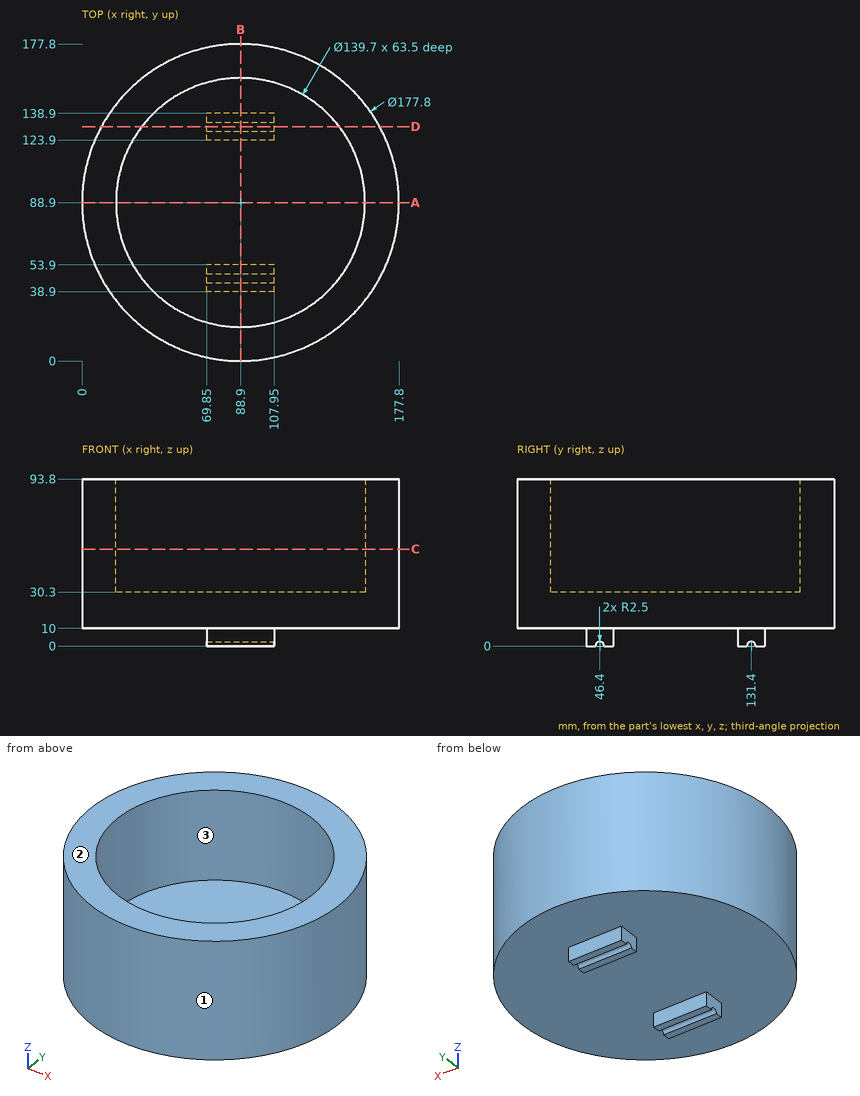
Here's the drawing with two shaded views (mm, measured from the low corner). I have some questions. Round coordinates to 2 decimals unless told otherwise and drop trailing zeros. Order: outer loops, then holes, each group sorted by start corner. A loop starts at its lowest first (then second) coordinate and runs counter-clockwise, first axis right, second up. Notation, with made-up numbers: (8, 89.25) -> (44, 89.25) arc R17 cw to (44, 99.25) -> close; hole circle Ø10 at (35.25, 23). An arc over 180 degrees is marked (long way). Use a Markdown table: item, result. Add a question column.
(1) Suppose I cut it at C-C, the plane z = 54.5. Please give me the cut outline in (x, y), and give its area (3 significant figures).
(2) Suppose I cut it at D-D, the plane y = 131.4. Please give me the cut outline in (x, z), and give its area (3 significant figures).
(3) Suppose I cut it at B-B, the plane x = 88.9. Please give me the cut outline in (y, z), and give its area (3 significant figures).
(4) I need wall thicknesses on line 1 along Y through (x, z) = (88, 62); line 2 along Z through (x, y) = (46.5, 43); line 3 along Y through (x, z) = (60, 79). Which ranges of each line are inside material? Lowest first, please.
(5) If we mould it in two halves opening along Y, with no side actions, what happens to the marked faces 1, 2 and 3? For each: released by +Y, released by -Y, zero draft, split by the parting line, or undercut.
(6) For pin 1 Ø8 at (y, z) = (44, 3) entering from -X; pin 2 Ø8 at (y, z) = (43, 3) entering from +X; pin 3 Ø6 at (x, y) = (129.5, 110) entering from +Z, each with a flat end and sliding along its axis, tell me the tip position at first contact or that it passes through.
(7) Suppose I cut it at A-A, the plane y = 88.9. Please give me the cut outline in (x, z), and give its area (3 significant figures).
Verdict:
| question | item | result |
|---|---|---|
| 1 | outline | circle Ø177.8 at (88.9, 88.9); hole circle Ø139.7 at (88.9, 88.9) |
| 1 | area | 9,500 mm2 |
| 2 | outline | (10.82, 10) -> (69.85, 10) -> (69.85, 2.5) -> (107.95, 2.5) -> (107.95, 10) -> (166.98, 10) -> (166.98, 93.8) -> (144.33, 93.8) -> (144.33, 30.3) -> (33.47, 30.3) -> (33.47, 93.8) -> (10.82, 93.8) -> close |
| 2 | area | 6,330 mm2 |
| 3 | outline | (0, 10) -> (38.9, 10) -> (38.9, 0) -> (43.9, 0) arc R2.5 cw to (48.9, 0) -> (53.9, 0) -> (53.9, 10) -> (123.9, 10) -> (123.9, 0) -> (128.9, 0) arc R2.5 cw to (133.9, 0) -> (138.9, 0) -> (138.9, 10) -> (177.8, 10) -> (177.8, 93.8) -> (158.75, 93.8) -> (158.75, 30.3) -> (19.05, 30.3) -> (19.05, 93.8) -> (0, 93.8) -> close |
| 3 | area | 6,310 mm2 |
| 4 | line 1 | 0 to 19.06, 158.74 to 177.8 |
| 4 | line 2 | 10 to 30.3 |
| 4 | line 3 | 4.83 to 25.31, 152.49 to 172.97 |
| 5 | face 1 | split by the parting line |
| 5 | face 2 | zero draft |
| 5 | face 3 | undercut |
| 6 | pin 1 | x = 69.85 |
| 6 | pin 2 | x = 107.95 |
| 6 | pin 3 | z = 30.3 |
| 7 | outline | (0, 10) -> (177.8, 10) -> (177.8, 93.8) -> (158.75, 93.8) -> (158.75, 30.3) -> (19.05, 30.3) -> (19.05, 93.8) -> (0, 93.8) -> close |
| 7 | area | 6,030 mm2 |
